```python
from build123d import *

# Parameters (mm, degrees)
CROQUIS1_W     = 5
CROQUIS1_H     = 7.4
EXTRUIR1_DEPTH = 0.75
EXTRUIR2_DEPTH = 5.5
CROQUIS3_W     = 5
CROQUIS3_H     = 4.9
EXTRUIR3_DEPTH = 4
CROQUIS4_R     = 2
EXTRUIR4_DEPTH = 6
CROQUIS5_R     = 0.5
EXTRUIR5_DEPTH = 2
CROQUIS6_R     = 0.45
EXTRUIR6_DEPTH = 3
EXTRUIR7_DEPTH = 0.1
CROQUIS8_R     = 0.385516529
EXTRUIR8_DEPTH = 0.1
EXTRUIR9_DEPTH = 0.1


with BuildPart() as part:
    # Croquis1 → Extruir1 (new, symmetric)
    with BuildSketch(Plane(origin=(0, 0, 0), x_dir=(0, 0, -1), z_dir=(1, 0, 0))):
        Rectangle(CROQUIS1_W, CROQUIS1_H)
    extrude(amount=EXTRUIR1_DEPTH, both=True)

    # Croquis2 → Extruir2 (add)
    with BuildSketch(Plane.ZY.offset(0.75)):
        with BuildLine():
            Line((-2.5, -3.7), (-2.5, 1.2))
            ThreePointArc((-2.5, 1.2), (0, 3.7), (2.5, 1.2))
            Line((2.5, 1.2), (2.5, -3.7))
            Line((2.5, -3.7), (-2.5, -3.7))
        make_face()
    extrude(amount=EXTRUIR2_DEPTH)

    # Croquis3 → Extruir3 (add)
    with BuildSketch(Plane.ZY.offset(6.25)):
        with Locations((0, -1.25)):
            Rectangle(CROQUIS3_W, CROQUIS3_H)
    extrude(amount=EXTRUIR3_DEPTH)

    # Croquis4 → Extruir4 (cut)
    with BuildSketch(Plane(origin=(0.75, 0, 0), x_dir=(0, 0, -1), z_dir=(1, 0, 0))):
        with Locations((0, 1.5)):
            Circle(CROQUIS4_R)
    extrude(amount=-EXTRUIR4_DEPTH, mode=Mode.SUBTRACT)

    # Croquis5 → Extruir5 (add)
    with BuildSketch(Plane(origin=(-5.25, 0, 0), x_dir=(0, 0, -1), z_dir=(1, 0, 0))):
        with Locations((0, 1.5)):
            Circle(CROQUIS5_R)
    extrude(amount=EXTRUIR5_DEPTH)

    # Croquis6 → Extruir6 (add)
    with BuildSketch(Plane(origin=(-3.25, 0, 0), x_dir=(0, 0, -1), z_dir=(1, 0, 0))):
        with Locations((0, 1.5)):
            Circle(CROQUIS6_R)
    extrude(amount=EXTRUIR6_DEPTH)

    # Croquis7 → Extruir7 (add)
    with BuildSketch(Plane.ZY.offset(10.25)):
        with BuildLine():
            Line((-1.5, -3.7), (-1.5, -0.3))
            ThreePointArc((-1.5, -0.3), (0, 1.2), (1.5, -0.3))
            Line((1.5, -0.3), (1.5, -3.7))
            Line((1.5, -3.7), (0.5, -3.7))
            Line((0.5, -3.7), (0.5, -4.7))
            ThreePointArc((0.5, -4.7), (0, -5.2), (-0.5, -4.7))
            Line((-0.5, -4.7), (-0.5, -3.7))
            Line((-0.5, -3.7), (-1.5, -3.7))
        make_face()
    extrude(amount=EXTRUIR7_DEPTH)

    # Croquis8 → Extruir8 (add)
    with BuildSketch(Plane.ZY.offset(10.35)):
        Circle(CROQUIS8_R)
    extrude(amount=EXTRUIR8_DEPTH)

    # Croquis9 → Extruir9 (add)
    with BuildSketch(Plane(origin=(0, 0, -2.5), x_dir=(-1, 0, 0), z_dir=(0, 0, -1))):
        Polygon((7.85, -3.7), (8.268709763, -4.118709763), (8.268709763, -5.1974269), (8.6, -5.528717137), (8.931290237, -5.1974269), (8.931290237, -4.118709763), (9.35, -3.7), (9.35, -1.3), (7.85, -1.3), align=None)
    extrude(amount=EXTRUIR9_DEPTH)


solid = part.part
```
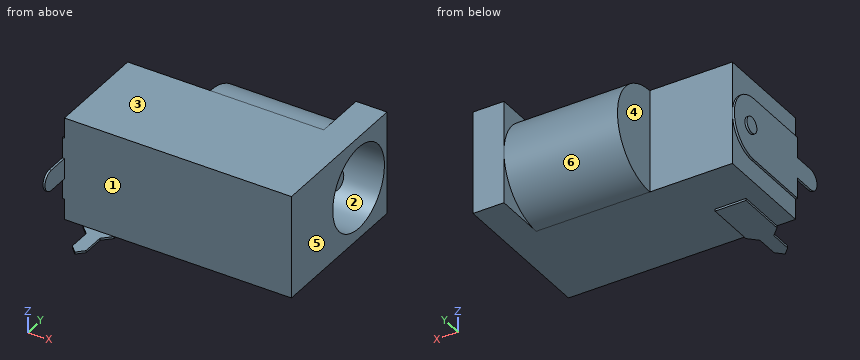
Input: part model. Units: mm. Frame: model coordinates. Face numbers are marked on the shaded views. A direction names the side the tool comes from. Coordinates: 2 decimals unless noted, no trailing zeros. Loops run counter-clockwise (first coordinate to the right, second up) from the corner with the lowest first, then second, coordinate; pieces in that order, holes last. Notation, with made-up numbers: M 50,-14 L 98,-14 A19 cw 98,5 Z; hole C 13,-36 d3. An arc over 180 degrees is marked long. Answer in a Markdown table with one row per item.
1. Section B-B, the plane y = 0. Output: boundary loops of the cut face in (x, z).
Response:
| item | result |
|---|---|
| outline | M -10.45,-0.39 L -10.35,-0.39 L -10.35,-1.47 L -10.25,-1.47 L -10.25,-2.5 L 0.75,-2.5 L 0.75,-1.32 L -5.25,-1.32 L -5.25,1.32 L 0.75,1.32 L 0.75,2.5 L -10.25,2.5 L -10.25,1.47 L -10.35,1.47 L -10.35,0.39 L -10.45,0.39 Z |
2. Section C-C, the plane z = -1.3. Output: boundary loops of the cut face in (x, y), then the cut area to 3 significant figures.
Response:
| item | result |
|---|---|
| outline | M -10.35,-3.7 L 0.75,-3.7 L 0.75,-0.02 L -5.25,-0.02 L -5.25,3.02 L 0.75,3.02 L 0.75,3.7 L -0.75,3.7 L -0.75,3.34 L -6.25,3.34 L -6.25,1.2 L -10.25,1.2 L -10.25,0.45 L -10.35,0.45 Z |
| area | 51.6 mm2 |
3. Draft query along Z for the marked faces 1, 2 and 3. Return one class per face: pulls with the +Z half, pulls with the -Z half, needs draft (parallel to the pull), parting line crosses it, or undercut.
Response:
| item | result |
|---|---|
| face 1 | needs draft |
| face 2 | undercut |
| face 3 | pulls with the +Z half |
4. Reachability of the marked faces 4, 5 and 6 from +Z, -Z, +X, -X, +Y, -Y: full face, straight path, thin tool, end or side. Return the list, or none.
Response:
| item | result |
|---|---|
| face 4 | +Z, -Z, -X, +Y |
| face 5 | +Z, -Z, +X, +Y, -Y |
| face 6 | -X, +Y |
5. Section A-A, the plane z = 2.15. Output: boundary loops of the cut face in (x, y).
Response:
| item | result |
|---|---|
| outline | M -10.25,-3.7 L 0.75,-3.7 L 0.75,3.7 L -0.75,3.7 L -0.75,2.48 L -6.25,2.48 L -6.25,1.2 L -10.25,1.2 Z |
6. Material intervals for line 1 (Y direction, x = -0.75, z = 0); line 2 (Y direction, x = -3.5, z = 0); line 3 (X direction, y = -0.5, z = -0.4), sorted ascending.
Response:
| item | result |
|---|---|
| line 1 | y = -3.7 to -0.5, 1.05 to 1.95, 3.5 to 3.7 |
| line 2 | y = -3.7 to -0.5, 1 to 2, 3.5 to 3.7 |
| line 3 | x = -10.35 to 0.75 |
7. First-contact query: pin 1 (1.5 mm diameter, centred on x = -5, y = -4.5, fed in from -Z); pin 2 (0.5 mm diameter, centred on y = -4.5, z = 0, fed in from +X); pin 3 (1.2 mm diameter, centred on y = 3, z = -1, fed in from -X); pin 4 (0.9 mm diameter, centred on y = -1.5, z = -0.5, fed in from -X). Flat tips, straight axial feed; report the tip coordinate or a pass-through.
Response:
| item | result |
|---|---|
| pin 1 | passes through |
| pin 2 | stops at x = -10.25 |
| pin 3 | stops at x = -6.25 |
| pin 4 | stops at x = -10.35 |
